```python
from build123d import *

# Parameters (mm, degrees)
BOX_W           = 50.8
BOX_H           = 476.25
BOX_DEPTH       = 50.8
BOX_PITCH_ANGLE = -20
THICKNESS_T     = -6.35


with BuildPart() as part:
    # Box → Box (new body)
    with BuildSketch(Plane.XY):
        with Locations((25.4, 238.125)):
            Rectangle(BOX_W, BOX_H)
    extrude(amount=BOX_DEPTH)


with BuildPart() as part_1:
    # Box pitch: moved
    add(part.part.rotate(Axis((0, 0, 0), (0, 1, 0)), BOX_PITCH_ANGLE))


with BuildPart() as part_2:
    # Box placement: moved
    add(part_1.part.moved(Location((866.852281, -479.425, 396.112887))))

    # Thickness
    thickness_openings = [part_2.faces().sort_by_distance(p)[0] for p in [
        (882.033162, -479.425, 428.668391),
        (882.033162, -3.175, 428.668391),
    ]]
    offset(amount=THICKNESS_T, openings=thickness_openings)


solid = part_2.part
```
Input: part model. Units: mm. Frame: model coordinates. A direction names the side the tool comes from. Give positions to 0.01 mm unless a question says otherwise; leave off trailing zeros. Order: outer loops, then holes, each group sorted by start corner. A loop starts at its lowest first (then second) coordinate and runs counter-clockwise, first axis right, second up.
1. Cut plane B-B (x = 884). Return loops of the section in (y, z) (3 decimals), and give its area (3 significant figures).
Computed:
outline: (-479.425, 402.354) - (-3.175, 402.354) - (-3.175, 409.112) - (-479.425, 409.112) - close; (-479.425, 449.657) - (-3.175, 449.657) - (-3.175, 456.414) - (-479.425, 456.414) - close
area: 6,440 mm2
2. Line query: probe 1 along X at (y, z) = (-175, 430); probe 2 along Z at (x, y) = (873, -318); probe 3 along X at (y, z) = (-189, 433.5). Output: solid intervals per line, ascending.
Computed:
probe 1: x = 854.52 to 861.28, 901.82 to 908.58
probe 2: z = 398.35 to 405.11, 445.65 to 452.41
probe 3: x = 853.24 to 860, 900.55 to 907.3
3. Pin query (flat end, axial travel): pin 1 Ø10 at (x, y) = (862.5, -113.5) entering from -Z; pin 2 Ø12 at (x, z) = (887, 445.5) entering from +Y (3 decimals); pin 3 Ø4 at (x, y) = (867.5, -368.5) entering from +Z; pin 4 Ø4 at (x, y) = (895.5, -232.5) entering from +Z. Return the tip coordinate at first contact, or that it passes through.
Computed:
pin 1: stops at z = 396.11
pin 2: stops at y = -3.175
pin 3: stops at z = 451.14
pin 4: stops at z = 461.22
4. Draft query along X for faces 3 (the face through (888.298, -237.966, 410.676)), 4 (the face through (890.39, -237.97, 404.68)), 5 (the face through (903, -3.175, 436)). Return one class per face: released by +X, released by -X, zero draft, split by the parting line, or undercut.
Computed:
face 3: undercut
face 4: released by +X
face 5: zero draft
5. Cut plane C-C (z = 434). Return loops of the section in (x, y) (1 decimal).
Computed:
outline: (853.1, -479.4) - (859.8, -479.4) - (859.8, -3.2) - (853.1, -3.2) - close; (900.4, -479.4) - (907.1, -479.4) - (907.1, -3.2) - (900.4, -3.2) - close
6. Set-up query: faces 1 (the face through (858.287, -244.634, 419.647)), 2 (the face through (875.27, -237.97, 446.48)). Return all of +Z, -Z, +X, -X, +Y, -Y with unobstructed straight access to the full face (end or side cutting, diameter ignored); none if empty.
Computed:
face 1: -Z, -X, +Y, -Y
face 2: +Y, -Y
7. Cut plane A-A (y = -266). Return loops of the section in (x, z), and give its area (3 significant figures).
Computed:
outline: (849.48, 443.85) - (866.85, 396.11) - (914.59, 413.49) - (897.21, 461.22) - close; hole (857.62, 440.05) - (870.65, 404.25) - (906.45, 417.28) - (893.42, 453.09) - close
area: 1,130 mm2
